For this review, use the dimensioned drawing (mm, ordinates from the lowest corner) and the shaded views. A direction names the side the tool comes from. Give positions to 0.01 mm unless a question says otherwise; leave off trailing zeros. Loops run counter-clockwise (first coordinate to the right, second up) from the corner with the lowest first, then second, coordinate; pieces in that order, holes last. Notation, with made-up numbers: (-5, 70) -> (26, 70) arc R12 cw to (26, 89) -> close; hole circle Ø1 at (22.25, 51.25). An arc over 180 degrees is marked (long way). Use a Markdown table: item, result. Add a question column.
1. Add section A-A (y = 393.5). State the section outline as (x, z) points (1 decimal).
2. For the marked faces 1, 2 and 3, list the 3-axis set-ups (+Z, -Z, +X, -X, +Y, -Y) from which the entire face can be reached by the end or side of a thin tool; tool diameter is ignored.
3. Draft analysis for pull direction X (two halves, no side actions). For the marked faces 4, 5, 6 and 7, state which applies: pulls with the +X half, pulls with the -X half, needs draft (parallel to the pull), parting line crosses it, or undercut.
4. To check wall thickness, follow line 1 (Y direction, x = 610.5, z = 525.5); line 2 (X direction, y = 216, z = 833); line 3 (Z direction, x = 53.5, y = 322) (1 decimal). State the ranges of each line that lie inside material, in increasing order.
5. Add section D-D (y = 136.5). State the section outline as (x, z) points.
6. For pin 1 Ø4 at (x, y) = (318, 208) entering from -Z (1 decimal); pin 2 Ø6 at (x, z) = (151, 1002.5) entering from -Y; pin 3 Ø1 at (y, z) = (56, 711.5) entering from -X (1 decimal), all flat-tipped, find the tip position at first contact; note any pin that passes through.
7. Add section B-B (x = 400). State the section outline as (y, z) points (1 decimal), and give its area (3 significant figures).
8. Add section C-C (z = 450.5). State the section outline as (x, y) points, and give its area (3 significant figures).
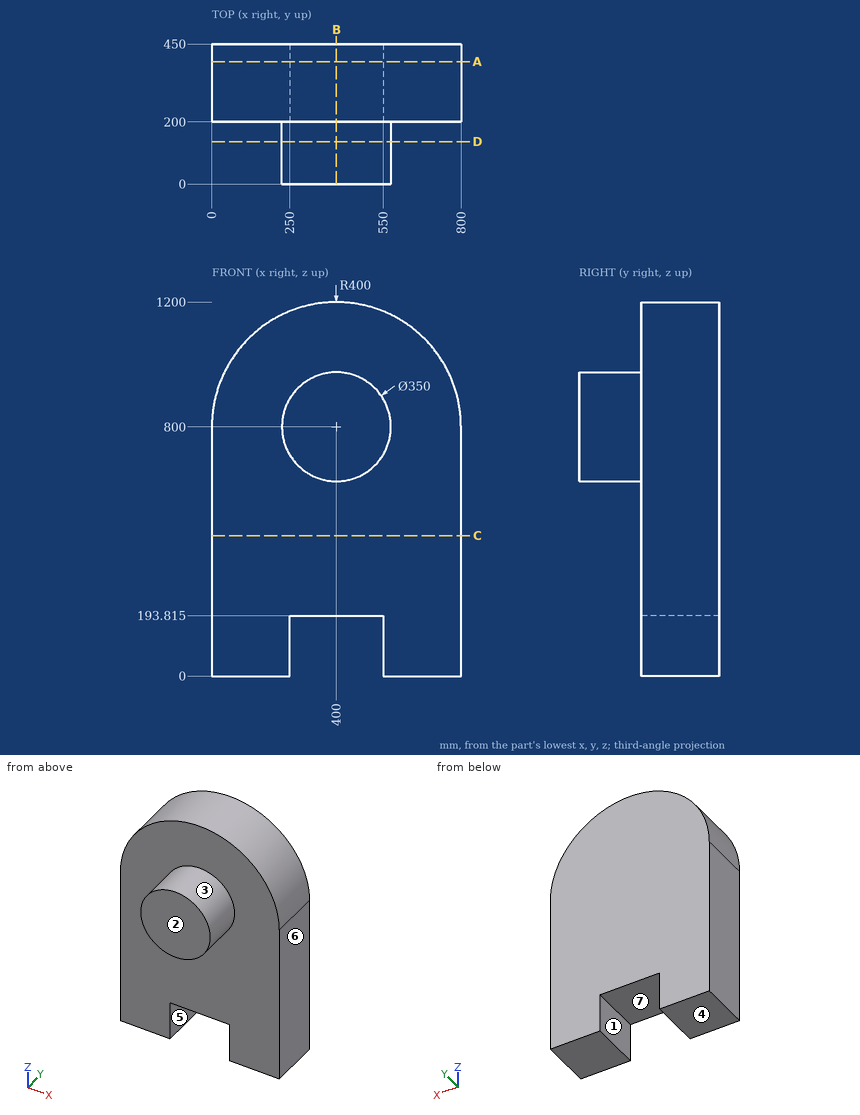
Taken from the geometry:
| question | item | result |
|---|---|---|
| 1 | outline | (0, 0) -> (250, 0) -> (250, 193.8) -> (550, 193.8) -> (550, 0) -> (800, 0) -> (800, 800) arc R400 ccw to (0, 800) -> close |
| 2 | face 1 | -Z, +Y, -Y |
| 2 | face 2 | +Z, -Z, +X, -X, -Y |
| 2 | face 3 | -Y |
| 3 | face 4 | needs draft |
| 3 | face 5 | undercut |
| 3 | face 6 | pulls with the +X half |
| 3 | face 7 | undercut |
| 4 | line 1 | y = 200 to 450 |
| 4 | line 2 | x = 1.36 to 798.64 |
| 4 | line 3 | z = 0 to 999.8 |
| 5 | outline | circle Ø350 at (400, 800) |
| 6 | pin 1 | stops at z = 193.8 |
| 6 | pin 2 | stops at y = 200 |
| 6 | pin 3 | stops at x = 248.7 |
| 7 | outline | (0, 625) -> (200, 625) -> (200, 193.8) -> (450, 193.8) -> (450, 1200) -> (200, 1200) -> (200, 975) -> (0, 975) -> close |
| 7 | area | 322,000 mm^2 |
| 8 | outline | (0, 200) -> (800, 200) -> (800, 450) -> (0, 450) -> close |
| 8 | area | 200,000 mm^2 |
